from build123d import *

# Parameters (mm, degrees)
SKETCH1_R               = 1.65
EXTRUDE1_DEPTH          = 6
SKETCH2_R               = 1.25
CUT_EXTRUDE1_DEPTH      = 4.55
SKETCH3_R               = 1.5
CUT_EXTRUDE2_DEPTH      = 4.5500001
CUT_EXTRUDE2_DEPTH_BACK = 3.25
CHAMFER1_SIZE           = 0.25


with BuildPart() as part:
    # Sketch1 → Extrude1 (new body, symmetric)
    with BuildSketch(Plane(origin=(0, 0, 0), x_dir=(0, 0, -1), z_dir=(1, 0, 0))):
        with BuildLine():
            Line((-2.225844711, 0.328808945), (-1.75, 3.55))
            Line((-1.75, 3.55), (1.75, 3.55))
            Line((1.75, 3.55), (2.225844711, 0.328808945))
            ThreePointArc((2.225844711, 0.328808945), (0, -2.25), (-2.225844711, 0.328808945))
        make_face()
        Circle(SKETCH1_R, mode=Mode.SUBTRACT)
    extrude(amount=EXTRUDE1_DEPTH, both=True)

    # Sketch2 → Cut-Extrude1 (cut, through all)
    with BuildSketch(Plane(origin=(0, 0, 0), x_dir=(1, 0, 0), z_dir=(0, 1, 0))):
        with Locations(Location((-4, 0, 0), (0, 0, 90))):  # turned: the seam where the file's is
            Circle(SKETCH2_R)
        with Locations(Location((4, 0, 0), (0, 0, 90))):  # turned: the seam where the file's is
            Circle(SKETCH2_R)
    extrude(amount=CUT_EXTRUDE1_DEPTH, mode=Mode.SUBTRACT)

    # Sketch3 → Cut-Extrude2 (cut, two sides)
    with BuildSketch(Plane(origin=(0, 0, 0), x_dir=(1, 0, 0), z_dir=(0, 1, 0))) as cut_extrude2_sk:
        with Locations(Location((0, 0, 0), (0, 0, 270))):  # turned: the seam where the file's is
            Circle(SKETCH3_R)
    extrude(amount=CUT_EXTRUDE2_DEPTH, mode=Mode.SUBTRACT)
    extrude(cut_extrude2_sk.sketch, amount=-CUT_EXTRUDE2_DEPTH_BACK, mode=Mode.SUBTRACT)

    # Chamfer1
    chamfer1_edges = [part.edges().sort_by_distance(p)[0] for p in [
        (-6, 0, 1.65),
        (6, 0, 1.65),
        (-4, 3.55, 1.25),
        (4, 3.55, 1.25),
    ]]
    chamfer(chamfer1_edges, length=CHAMFER1_SIZE)


solid = part.part
Verification items for the finished model (mm, model axes). A direction names the side the tool comes from. Give positions to 0.01 mm unless a question says otherwise; leave off trailing zeros. Write each loop counter-clockwise with the first axis right and the second up, starting at its lowest first coordinate (ties: lowest second). Pieces come first, ordered by that corner, then holes. Notation, with made-up numbers: (15.5, -19) - (22.5, -19) arc R15 cw to (22.5, -5) - close; hole circle Ø4 at (15.5, 16). An arc over 180 degrees is marked (long way). Answer as CSV lines item,"result". Start each with the question number.
1. Set-up check for faces 5 (the face through (-3.521, 2.42, -1.155)), 6 (the face through (-6, 2, 0.5)): record each of +Z, -Z, +X, -X, +Y, -Y from which the full face is reachable in a straight line by a thin tool's end or side.
2. Thickness scan on line 1 (X direction, y = 2.75, z = 0); line 2 (X direction, y = 1.7, z = 0); line 3 (Z direction, x = -3, y = 0.65). Record the ranges inside material, lowest first.
3. Depth check by flat-ended pin: pin 1 (1.5 mm diameter, centred on x = -2, z = -2, fed in from -Y); pin 2 (3 mm diameter, centred on x = 4, y = 2.5, fed in from +Z); pin 3 (2 mm diameter, centred on x = -3, y = -0.5, fed in from -Z); pin 4 (1.5 mm diameter, centred on x = -4, z = 0, fed in from +Y). Enter the tip coordinate at first touch or a pass-through.
4. Sectioned sample at C-C (x = 0). Record the boundary of the cut face in (y, z).
5. Sectioned sample at B-B (z = 0). Count the separate pieces of the cut face and the enclosed holes in it, then the cut area to 4 significant figures.
6. Sectioned sample at D-D (x = -4). Record the boundary of the cut face in (y, z), then the cut area to 3 significant figures.
7. Draft check along Z on faces 1 (the face through (0.08, 1.92, 1.99)), 2 (the face through (4.479, 2.42, -1.155)), 3 (the face through (0.084, 1.962, -1.985)), 4 (the face through (-0.08, 0.496, -1.574)). Enter one of: pulls with the +Z half, pulls with the -Z half, needs draft (parallel to the pull), parting line crosses it, or undercut.
8. Sectioned sample at A-A (y = 0). Record the boundary of the cut face in (x, z), then the cut area to 3 significant figures.
Derived:
1,face 5,"+Y"
1,face 6,"+Z, -Z, -X, +Y, -Y"
2,line 1,"-6 to -5.25, -2.75 to -1.5, 1.5 to 2.75, 5.25 to 6"
2,line 2,"-5.8 to -5.25, -2.75 to -1.5, 1.5 to 2.75, 5.25 to 5.8"
2,line 3,"-2.18 to -1.52, 1.52 to 2.18"
3,pin 1,"y = -1.87"
3,pin 2,"z = 2.13"
3,pin 3,"z = -2.25"
3,pin 4,"y = -1.47"
4,outline,"(-1.68, -1.5) arc R2.25 ccw to (0.33, -2.23) - (3.55, -1.75) - (3.55, -1.5) - (0.69, -1.5) arc R1.65 cw to (-0.69, -1.5) - close; (-1.68, 1.5) - (-0.69, 1.5) arc R1.65 cw to (0.69, 1.5) - (3.55, 1.5) - (3.55, 1.75) - (0.33, 2.23) arc R2.25 ccw to start"
5,separate pieces,"6"
5,enclosed holes,"0"
5,area,"12.75 mm²"
6,outline,"(0.33, -2.23) - (3.55, -1.75) - (3.55, -1.5) - (3.3, -1.25) - (1.08, -1.25) arc R1.65 cw (long way) to (1.08, 1.25) - (3.3, 1.25) - (3.55, 1.5) - (3.55, 1.75) - (0.33, 2.23) arc R2.25 ccw (long way) to start"
6,area,"8.43 mm²"
7,face 1,"pulls with the +Z half"
7,face 2,"undercut"
7,face 3,"pulls with the -Z half"
7,face 4,"undercut"
8,outline,"(-6, -2.25) - (6, -2.25) - (6, -1.9) - (5.75, -1.65) - (-5.75, -1.65) - (-6, -1.9) - close; (-6, 1.9) - (-5.75, 1.65) - (5.75, 1.65) - (6, 1.9) - (6, 2.25) - (-6, 2.25) - close"
8,area,"14.3 mm²"
